Work out the finished part from the listing and answer in its coordinate system (mm). A direction names the side the tool comes from. Round coordinates to 2 decimals unless told otherwise and drop trailing zeros. Loops run counter-clockwise (first coordinate to the right, second up) from the corner with the lowest first, then second, coordinate; pieces in that order, holes last.
```python
from build123d import *

# Parameters (mm, degrees)
SALIENTE_EXTRUIR2_DEPTH   = 46.5
CROQUIS3_R                = 1.500774296
CROQUIS3_R_2              = 1.503322105
CORTAR_EXTRUIR1_DEPTH     = 46.5
CORTAR_EXTRUIR2_START     = 16.5
CORTAR_EXTRUIR2_OUTLINE_R = 1.500774296
CORTAR_EXTRUIR2_DEPTH     = 30
REDONDEO2_R               = 3
CORTAR_EXTRUIR3_START     = -46.5
CORTAR_EXTRUIR3_OUTLINE_R = 1.500774296
CORTAR_EXTRUIR3_DEPTH     = 30
REDONDEO3_R               = 3
CORTAR_EXTRUIR4_START     = 10
CORTAR_EXTRUIR4_OUTLINE_R = 1.503322105
CORTAR_EXTRUIR4_DEPTH     = 20
CORTAR_EXTRUIR5_START     = -27
CORTAR_EXTRUIR5_OUTLINE_R = 1.503322105
CORTAR_EXTRUIR5_DEPTH     = 17
REDONDEO4_R               = 1
CROQUIS4_W                = 18.6
CROQUIS4_H                = 6
CORTAR_EXTRUIR6_DEPTH     = 133.823646461
CROQUIS5_W                = 18.6
CROQUIS5_H                = 6
CORTAR_EXTRUIR7_DEPTH     = 133.823646461
REDONDEO5_R               = 1.5
REDONDEO6_R               = 2


# Read off the part's stored shape, not the designer's step: Cortar-Extruir2, Cortar-Extruir3, Cortar-Extruir4, Cortar-Extruir5
with BuildPart() as part:
    # Croquis1 → Saliente-Extruir2 (new, symmetric)
    with BuildSketch(Plane.XY):
        with BuildLine():
            Line((-10.68367701, -0.137920216), (-8.740480313, -4.5))
            Line((-8.740480313, -4.5), (39, -4.5))
            Line((39, -4.5), (39, -10.5))
            Line((39, -10.5), (-26, -10.5))
            Line((-26, -10.5), (-26, -26.1))
            Line((-26, -26.1), (-30, -26.1))
            Line((-30, -26.1), (-30, -10.5))
            Line((-30, -10.5), (-81.2, -10.5))
            ThreePointArc((-81.2, -10.5), (-82.649747468, -7), (-81.2, -3.5))
            Line((-81.2, -3.5), (-68.491106331, 8.777732226))
            ThreePointArc((-68.491106331, 8.777732226), (-65.272311444, 9.670901246), (-62.770376094, 7.457598075))
            Line((-62.770376094, 7.457598075), (-58.782136556, -3.5))
            Line((-58.782136556, -3.5), (-29.179236041, -3.5))
            Line((-29.179236041, -3.5), (-22.771154479, -2.137920216))
            ThreePointArc((-22.771154479, -2.137920216), (-21.470497358, 3.176104142), (-16.576957377, 0.729917256))
            ThreePointArc((-16.576957377, 0.729917256), (-13.638551951, 0.240078221), (-10.68367701, -0.137920216))
        make_face()
    extrude(amount=SALIENTE_EXTRUIR2_DEPTH, both=True)

    # Croquis3 → Cortar-Extruir1 (cut, symmetric)
    with BuildSketch(Plane.XY):
        with Locations((-66.059300267, 6.260527573)):
            Circle(CROQUIS3_R)
        with Locations((-20, 0)):
            Circle(CROQUIS3_R_2)
    extrude(amount=CORTAR_EXTRUIR1_DEPTH, both=True, mode=Mode.SUBTRACT)

    # Cortar-Extruir2 outline → Cortar-Extruir2 (cut)
    with BuildSketch(Plane.XY.offset(CORTAR_EXTRUIR2_START)):
        with BuildLine():
            Line((-68.491106331, 8.777732226), (-69.201699105, 8.091246996))
            ThreePointArc((-69.201699105, 8.091246996), (-66.848168988, 2.721235528), (-62.462991688, 6.61306636))
            Line((-62.462991688, 6.61306636), (-62.770376094, 7.457598075))
            ThreePointArc((-62.770376094, 7.457598075), (-65.272311444, 9.670901246), (-68.491106331, 8.777732226))
        make_face()
        with Locations((-66.059300267, 6.260527573)):
            Circle(CORTAR_EXTRUIR2_OUTLINE_R, mode=Mode.SUBTRACT)
    extrude(amount=CORTAR_EXTRUIR2_DEPTH, mode=Mode.SUBTRACT)

    # Redondeo2
    redondeo2_edges = [part.edges().sort_by_distance(p)[0] for p in [
        (-62.462991688, 6.61306636, 31.5),
    ]]
    fillet(redondeo2_edges, radius=REDONDEO2_R)

    # Cortar-Extruir3 outline → Cortar-Extruir3 (cut)
    with BuildSketch(Plane.XY.offset(CORTAR_EXTRUIR3_START)):
        with BuildLine():
            ThreePointArc((-69.164573514, 8.127113066), (-66.827048097, 2.685630168), (-62.508602445, 6.738380883))
            Line((-62.508602445, 6.738380883), (-62.770376094, 7.457598075))
            ThreePointArc((-62.770376094, 7.457598075), (-65.272311444, 9.670901246), (-68.491106331, 8.777732226))
            Line((-68.491106331, 8.777732226), (-69.164573514, 8.127113066))
        make_face()
        with Locations((-66.059300267, 6.260527573)):
            Circle(CORTAR_EXTRUIR3_OUTLINE_R, mode=Mode.SUBTRACT)
    extrude(amount=CORTAR_EXTRUIR3_DEPTH, mode=Mode.SUBTRACT)

    # Redondeo3
    redondeo3_edges = [part.edges().sort_by_distance(p)[0] for p in [
        (-62.508602445, 6.738380883, -31.5),
    ]]
    fillet(redondeo3_edges, radius=REDONDEO3_R)

    # Cortar-Extruir4 outline → Cortar-Extruir4 (cut)
    with BuildSketch(Plane.XY.offset(CORTAR_EXTRUIR4_START)):
        with BuildLine():
            Line((-22.771154479, -2.137920216), (-22.827271519, -2.149848262))
            ThreePointArc((-22.827271519, -2.149848262), (-18.523452571, -3.240720775), (-16.513304708, 0.718087877))
            ThreePointArc((-16.513304708, 0.718087877), (-16.545132262, 0.723996005), (-16.576957377, 0.729917256))
            ThreePointArc((-16.576957377, 0.729917256), (-21.470497358, 3.176104142), (-22.771154479, -2.137920216))
        make_face()
        with Locations((-20, 0)):
            Circle(CORTAR_EXTRUIR4_OUTLINE_R, mode=Mode.SUBTRACT)
    extrude(amount=CORTAR_EXTRUIR4_DEPTH, mode=Mode.SUBTRACT)

    # Cortar-Extruir5 outline → Cortar-Extruir5 (cut)
    with BuildSketch(Plane.XY.offset(CORTAR_EXTRUIR5_START)):
        with BuildLine():
            ThreePointArc((-22.813751372, -2.146974465), (-18.533466696, -3.203987987), (-16.523253553, 0.719933216))
            ThreePointArc((-16.523253553, 0.719933216), (-16.550106333, 0.724920565), (-16.576957377, 0.729917256))
            ThreePointArc((-16.576957377, 0.729917256), (-21.470497358, 3.176104142), (-22.771154479, -2.137920216))
            Line((-22.771154479, -2.137920216), (-22.813751372, -2.146974465))
        make_face()
        with Locations((-20, 0)):
            Circle(CORTAR_EXTRUIR5_OUTLINE_R, mode=Mode.SUBTRACT)
    extrude(amount=CORTAR_EXTRUIR5_DEPTH, mode=Mode.SUBTRACT)

    # Redondeo4
    redondeo4_edges = [part.edges().sort_by_distance(p)[0] for p in [
        (-69.201699105, 8.091246996, 31.5),
        (-69.164573514, 8.127113066, -31.5),
    ]]
    fillet(redondeo4_edges, radius=REDONDEO4_R)

    # Croquis4 → Cortar-Extruir6 (cut, through all)
    with BuildSketch(Plane(origin=(39, 0, 0), x_dir=(0, 0, -1), z_dir=(1, 0, 0))):
        with Locations((18.6, -7.5)):
            Rectangle(CROQUIS4_W, CROQUIS4_H)
    extrude(amount=-CORTAR_EXTRUIR6_DEPTH, mode=Mode.SUBTRACT)

    # Croquis5 → Cortar-Extruir7 (cut, through all)
    with BuildSketch(Plane(origin=(39, 0, 0), x_dir=(0, 0, -1), z_dir=(1, 0, 0))):
        with Locations((-18.6, -7.5)):
            Rectangle(CROQUIS5_W, CROQUIS5_H)
    extrude(amount=-CORTAR_EXTRUIR7_DEPTH, mode=Mode.SUBTRACT)

    # Redondeo5
    redondeo5_edges = [part.edges().sort_by_distance(p)[0] for p in [
        (39, -4.5, -37.2),
        (15.129759844, -4.5, -46.5),
        (39, -10.5, -37.2),
        (39, -7.5, -46.5),
        (6.5, -10.5, -46.5),
        (6.5, -10.5, -27.9),
        (15.129759844, -4.5, -27.9),
        (6.5, -10.5, -9.3),
        (15.129759844, -4.5, -9.3),
        (39, -7.5, -27.9),
        (39, -7.5, -9.3),
        (39, -4.5, 0),
        (39, -10.5, 0),
        (6.5, -10.5, 9.3),
        (15.129759844, -4.5, 9.3),
        (6.5, -10.5, 27.9),
        (15.129759844, -4.5, 27.9),
        (39, -7.5, 9.3),
        (39, -7.5, 27.9),
        (39, -4.5, 37.2),
        (39, -10.5, 37.2),
        (6.5, -10.5, 46.5),
        (39, -7.5, 46.5),
        (15.129759844, -4.5, 46.5),
    ]]
    fillet(redondeo5_edges, radius=REDONDEO5_R)

    # Redondeo6
    redondeo6_edges = [part.edges().sort_by_distance(p)[0] for p in [
        (-10.68367701, -0.137920216, 0),
    ]]
    fillet(redondeo6_edges, radius=REDONDEO6_R)


solid = part.part
```
1. Find section D-D (y = -19). Write down the section's boundary in (x, z).
Answer key:
outline: (-30, -46.5) - (-26, -46.5) - (-26, 46.5) - (-30, 46.5) - close
2. Find section C-C (x = -38). Write down the section's boundary in (y, z), then the cut area to 3 significant figures.
Answer key:
outline: (-10.5, -46.5) - (-3.5, -46.5) - (-3.5, 46.5) - (-10.5, 46.5) - (-10.5, 27.9) - (-4.5, 27.9) - (-4.5, 9.3) - (-10.5, 9.3) - (-10.5, -9.3) - (-4.5, -9.3) - (-4.5, -27.9) - (-10.5, -27.9) - close
area: 428 mm2
3. Given pin 1 (12.5 mm diameter, centred on x = 13, z = -35, fed in from -Y); pin 2 (17 mm diameter, centred on x = 20, z = -1.5, fed in from +Y); pin 3 (2.5 mm diameter, centred on x = -68, y = 6.5, fed in from -Z); pin 4 (4 mm diameter, centred on x = -2, y = -5.5, fed in from -Z), each flat-ended and moving along its own axis, determine where each tip first touches the part or whether it passes through.
Answer key:
pin 1: stops at y = -10.5
pin 2: stops at y = -4.5
pin 3: stops at z = -16.5
pin 4: stops at z = -46.5
4. Consider probe 1 along Z at (x, y) = (-47.5, -7); probe 2 along Y at (x, z) = (-20, 4.75); probe 3 along Y at (x, z) = (17, -37). Determine where each line is inside the solid, lowest interval first.
Answer key:
probe 1: z = -46.5 to -27.9, -9.3 to 9.3, 27.9 to 46.5
probe 2: y = -10.5 to -1.5, 1.5 to 3.5
probe 3: y = -10.5 to -4.5
5. Which of the six approach directions +Z, -Z, +X, -X, +Y, -Y give full straight-line access (tool end or side, diameter ignored) to faces 4 (the face through (-67.762, 3.055, 31.29)), 5 (the face through (-76.347, 1.189, 0.651)), 6 (the face through (14, -4.5, -37)), 7 (the face through (-55, -10.5, 0)), 8 (the face through (-36, -6, -46.5))?
Answer key:
face 4: +Z, +Y
face 5: +Z, -Z, -X, +Y
face 6: +Z, -Z, +X, +Y
face 7: +Z, -Z, -X, -Y
face 8: -Z, +X, -X, +Y, -Y
6. Find section A-A (x = 16.5). Write down the section's boundary in (y, z), then the cut area to 3 significant figures.
Answer key:
outline: (-10.5, -45) arc R1.5 ccw to (-9, -46.5) - (-6, -46.5) arc R1.5 ccw to (-4.5, -45) - (-4.5, -29.4) arc R1.5 ccw to (-6, -27.9) - (-9, -27.9) arc R1.5 ccw to (-10.5, -29.4) - close; (-10.5, -7.8) arc R1.5 ccw to (-9, -9.3) - (-6, -9.3) arc R1.5 ccw to (-4.5, -7.8) - (-4.5, 7.8) arc R1.5 ccw to (-6, 9.3) - (-9, 9.3) arc R1.5 ccw to (-10.5, 7.8) - close; (-10.5, 29.4) arc R1.5 ccw to (-9, 27.9) - (-6, 27.9) arc R1.5 ccw to (-4.5, 29.4) - (-4.5, 45) arc R1.5 ccw to (-6, 46.5) - (-9, 46.5) arc R1.5 ccw to (-10.5, 45) - close
area: 329 mm2
7. Determine the mould class of faces 1 (the face through (-66, 4.6, -16.5)), 2 (the face through (-45, -4.5, 19)), 3 (the face through (-62.14, 2.97, -31.29)) for opening direction Z: +Z half, -Z half, draft (parallel to the pull), parting line (faces both ways), or undercut.
Answer key:
face 1: -Z half
face 2: undercut
face 3: draft
8. Find section B-B (z = 24). Write down the section's boundary in (x, y).
Answer key:
outline: (-81.97, -4.5) - (-8.74, -4.5) - (-10.22, -1.18) arc R2 ccw to (-11.8, -0.01) arc R78.5 cw to (-16.51, 0.72) arc R3.55 cw to (-22.83, -2.15) - (-29.18, -3.5) - (-58.78, -3.5) - (-60.51, 1.26) arc R3 ccw to (-64.57, 2.96) arc R3.63 cw to (-69.62, 5.54) arc R1 ccw to (-71.3, 6.06) - (-81.2, -3.5) arc R4.95 ccw to start; (-30, -26.1) - (-26, -26.1) - (-26, -10.5) - (-30, -10.5) - close
